Can you work these out from the model? Positions are in its coordinate system, mm. Round coordinates to 2 decimals unless told otherwise and drop trailing zeros. Loops run counter-clockwise (first coordinate to the right, second up) from the corner with the lowest first, then second, coordinate; pieces in that order, holes last.
(1) Will these pins go through, and if not, where does the flat tip stop? pin 1 Ø5 at (x, y) = (-8.5, -97.5) entering from +Z; pin 2 Ø0.5 at (x, z) = (-25.5, 4) entering from -Y; pin 3 Ø2 at (y, z) = (-155.5, 2.5) entering from +X.
(2) I want a section at B-B on x = 1. Write out the boundary of the cut face in (y, z), plus the area to 3 significant figures.
(3) I want a section at D-D on y = -174. Write out the boundary of the cut face in (x, z).
(4) I want a section at A-A on z = 1.7. Write out the boundary of the cut face in (x, y), plus the area to 3 significant figures.
(5) I want a section at C-C on y = -77.5. Write out the boundary of the cut face in (x, z), plus the area to 3 significant figures.
(6) If I drill on line 1 along X through (y, z) = (-97.5, 0.9); line 2 along Y through (x, z) = (0, 1); line 3 along Z through (x, y) = (-30, -87.5), over which ranges is the centre line in solid material (lowest first)?
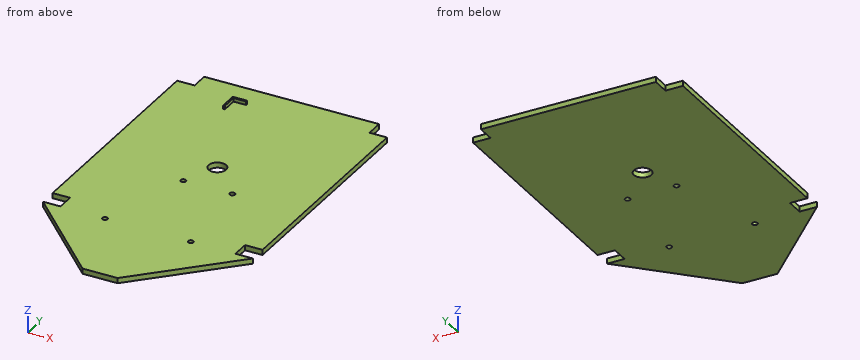
from build123d import *

# Parameters (mm, degrees)
EXTRUSION1_DEPTH        = 3
ESQUISSE2_R             = 1.5
ENL_V_MAT_EXTRU_1_DEPTH = 10
EXTRUSION2_DEPTH        = 2
ESQUISSE4_R             = 5
ENL_V_MAT_EXTRU_2_DEPTH = 52


with BuildPart() as part:
    # Esquisse1 → Extrusion1 (new body)
    with BuildSketch(Plane.XY):
        Polygon((50, 0), (-50, 0), (-50, -10), (-60, -10), (-60, -140), (-50, -140), (-50, -150), (-60, -150), (-10, -200), (10, -200), (60, -150), (50, -150), (50, -140), (60, -140), (60, -10), (50, -10), align=None)
    extrude(amount=EXTRUSION1_DEPTH)

    # Esquisse2 → Enlèv. mat.-Extru.1 (cut)
    with BuildSketch(Plane.XY.offset(3)):
        with Locations((-24.5, -150)):
            Circle(ESQUISSE2_R)
        with Locations((-8.5, -97.5)):
            Circle(ESQUISSE2_R)
        with Locations((19.5, -97.5)):
            Circle(ESQUISSE2_R)
        with Locations((24.5, -150)):
            Circle(ESQUISSE2_R)
    extrude(amount=-ENL_V_MAT_EXTRU_1_DEPTH, mode=Mode.SUBTRACT)

    # Esquisse3 → Extrusion2 (add)
    with BuildSketch(Plane.XY.offset(3)):
        Polygon((-25, -15), (-25, -24.03748446), (-26, -24.03748446), (-26, -14), (-17.773776224, -14), (-17.773776224, -15), align=None)
    extrude(amount=EXTRUSION2_DEPTH)

    # Esquisse4 → Enlèv. mat.-Extru.2 (cut)
    with BuildSketch(Plane.XY.offset(3)):
        with Locations((0, -77.5)):
            Circle(ESQUISSE4_R)
    extrude(amount=-ENL_V_MAT_EXTRU_2_DEPTH, mode=Mode.SUBTRACT)


solid = part.part
Filled sheet:
1. pin 1: stops at z = 3
1. pin 2: stops at y = -24.04
1. pin 3: stops at x = 55.5
2. outline: (-200, 0) - (-82.4, 0) - (-82.4, 3) - (-200, 3) - close; (-72.6, 0) - (0, 0) - (0, 3) - (-72.6, 3) - close
2. area: 571 mm2
3. outline: (-36, 0) - (36, 0) - (36, 3) - (-36, 3) - close
4. outline: (-60, -150) - (-10, -200) - (10, -200) - (60, -150) - (50, -150) - (50, -140) - (60, -140) - (60, -10) - (50, -10) - (50, 0) - (-50, 0) - (-50, -10) - (-60, -10) - (-60, -140) - (-50, -140) - (-50, -150) - close; hole circle Ø3 at (-24.5, -150); hole circle Ø3 at (-8.5, -97.5); hole circle Ø10 at (0, -77.5); hole circle Ø3 at (19.5, -97.5); hole circle Ø3 at (24.5, -150)
4. area: 21,000 mm2
5. outline: (-60, 0) - (-5, 0) - (-5, 3) - (-60, 3) - close; (5, 0) - (60, 0) - (60, 3) - (5, 3) - close
5. area: 330 mm2
6. line 1: x = -60 to -10, -7 to 18, 21 to 60
6. line 2: y = -200 to -82.5, -72.5 to 0
6. line 3: z = 0 to 3
